Source: three-view drawing plus pictorial views. Frame: mm from the lowest corner of the part. A direction names the side the tool comes from. Give positions to 0.01 mm unless a question says otherwise; leave off trailing zeros. Order: outer loops, then holes, each group sorted by start corner. A loop starts at its lowest first (then second) coordinate and runs counter-clockwise, first axis right, second up. Notation, with made-up numbers: (27.25, 37.25) - (46.25, 37.25) arc R17 ccw to (46.25, 60.25) - close; hole circle Ø2 at (86.5, 60.25). An arc over 180 degrees is marked (long way). Use one line per item in the form item = value.
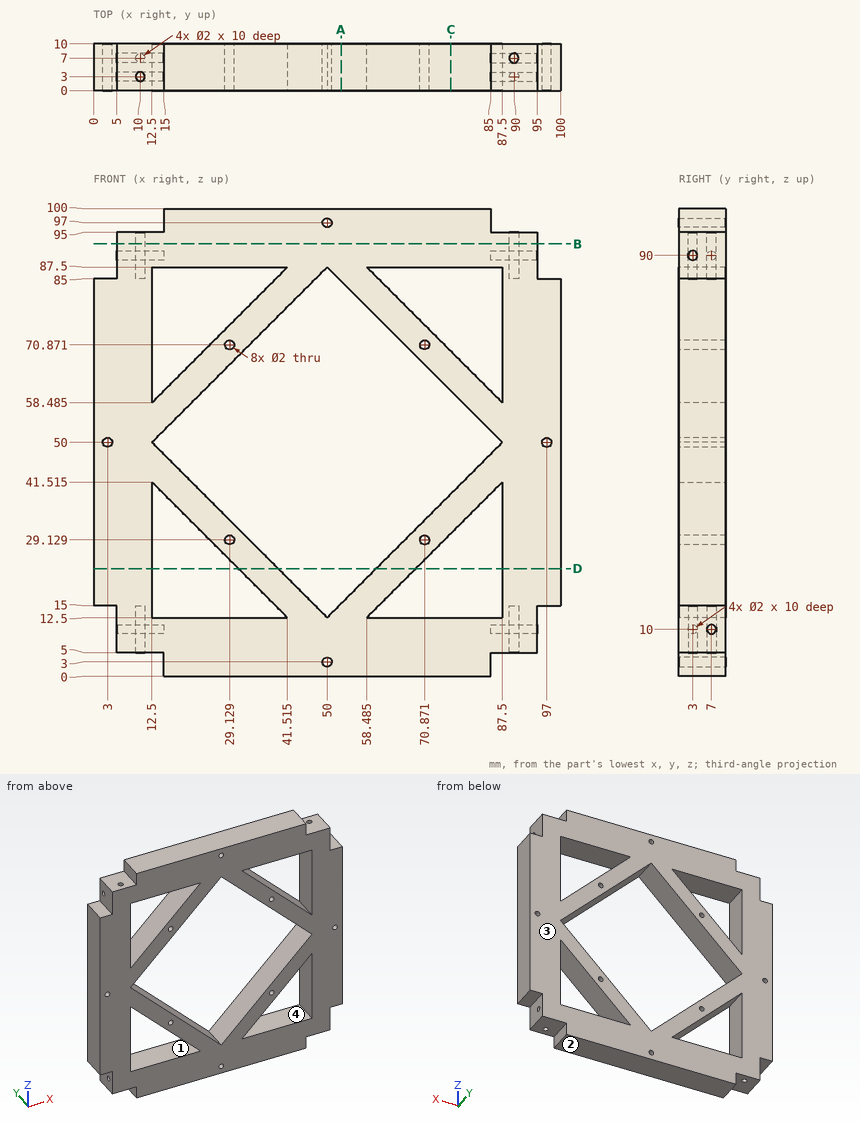
(1) Pull-direction query (X, two-part tool) for the marked faces 3 and 4; classes: released by +X, released by -X, zero draft, split by the parting line, or undercut.
Computed values:
face_3 = zero draft
face_4 = undercut
(2) Contact query for flat-ended pins moving along their axis: pin 1 Ø2.5 at (y, z) = (7, 90) entering from +X; pin 2 Ø1.6 at (x, y) = (10.5, 3.5) entering from +Z; pin 3 Ø5.5 at (y, z) = (5.5, 98.5) entering from -X; pin 4 Ø1.6 at (x, z) = (29.13, 70.87) entering from -Y (1 decimal). Output: stop coordinate, or through.
Computed values:
pin_1 = 95
pin_2 = 95
pin_3 = 15
pin_4 = through
(3) Cut plane D-D on z = 23. Output: boundary loops of the cut face in (x, y) (1 decimal).
Computed values:
outline = (0, 0) - (12.5, 0) - (12.5, 10) - (0, 10) - close; (31, 0) - (39.5, 0) - (39.5, 10) - (31, 10) - close; (60.5, 0) - (69, 0) - (69, 10) - (60.5, 10) - close; (87.5, 0) - (100, 0) - (100, 10) - (87.5, 10) - close
(4) Reachability of the marked faces 1 and 2 from +Z, -Z, +X, -X, +Y, -Y: full face, straight path, thin tool, end or side. Return the list, or none.
Computed values:
face_1 = +Y, -Y
face_2 = -Z, +X, -X, +Y, -Y
(5) Cut plane A-A on x = 53. Output: boundary loops of the cut face in (y, z).
Computed values:
outline = (0, 0) - (10, 0) - (10, 15.5) - (0, 15.5) - close; (0, 84.5) - (10, 84.5) - (10, 100) - (0, 100) - close
(6) Cut plane B-B on z = 92.5. Output: boundary loops of the cut face in (x, y), plus the area to 3 significant figures.
Computed values:
outline = (5, 0) - (95, 0) - (95, 10) - (5, 10) - close; hole circle Ø2 at (10, 3); hole circle Ø2 at (90, 7)
area = 894 mm²
(7) Cut plane C-C on x = 76.5. Output: boundary loops of the cut face in (y, z) (1 decimal), plus the area to 3 significant figures.
Computed values:
outline = (0, 0) - (10, 0) - (10, 12.5) - (0, 12.5) - close; (0, 30.5) - (10, 30.5) - (10, 39) - (0, 39) - close; (0, 61) - (10, 61) - (10, 69.5) - (0, 69.5) - close; (0, 87.5) - (10, 87.5) - (10, 100) - (0, 100) - close
area = 420 mm²
(8) Ray query, line 1 along X through (y, z) = (3.5, 3); line 2 along Y through (x, z) = (10, 88); line 3 along X through (y, z) = (2.25, 35) (1 decimal). Return the intervals inside material, ascending.
Computed values:
line_1 = 15 to 49, 51 to 85
line_2 = 0 to 2, 4 to 10
line_3 = 0 to 12.5, 19 to 27.5, 72.5 to 81, 87.5 to 100
